Geometry check sheet. Reference: drawing and pictorial views, mm from the part's lowest x, y, z. Give positions to 0.01 mm unless a question says otherwise; leave off trailing zeros. Write each loop counter-clockwise with the first axis right and the second up, starting at its lowest first coordinate (ties: lowest second). Pieces come first, ordered by that corner, then holes. Notation, with made-up numbers: (-14, -12) - (35, -12) arc R6 ccw to (35, -3) - close; hole circle Ø9 at (2.25, 45.25). An arc over 180 degrees is marked (long way). Put each result on its own line as item: value.
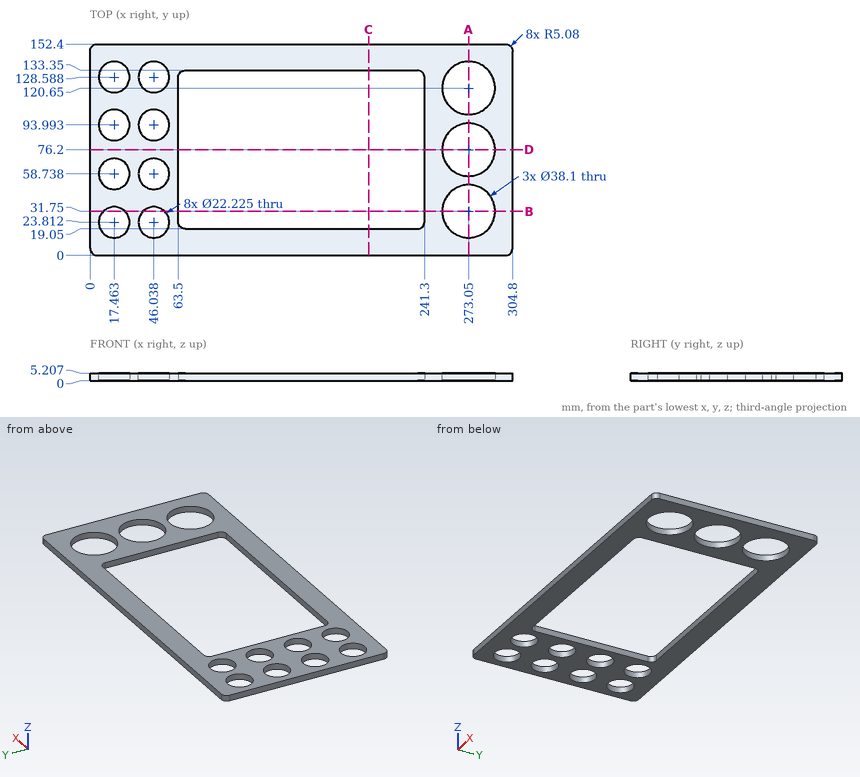
Q1. Section check D-D, the plane y = 76.2. Record the cut outline in (x, z), plus the area to 3 significant figures.
Answers follow:
outline: (0, 0) - (63.5, 0) - (63.5, 5.21) - (0, 5.21) - close; (241.3, 0) - (254, 0) - (254, 5.21) - (241.3, 5.21) - close; (292.1, 0) - (304.8, 0) - (304.8, 5.21) - (292.1, 5.21) - close
area: 463 mm2
Q2. Go/stop test with a flat-tipped pin: pin 1 Ø13.5 at (x, y) = (46.04, 23.81) entering from +Z. Record where the tip stops, or that it passes through.
Answers follow:
pin 1: passes through
Q3. Scan lines: line 1 along X through (y, z) = (25, 1.35) (1 decimal); line 2 along Y through (x, z) = (207.5, 2); line 3 along Y through (x, z) = (43, 1.45). Record each from-to range of solid material in increasing order.
Answers follow:
line 1: x = 0 to 6.4, 28.5 to 35, 57.1 to 63.5, 241.3 to 255.2, 290.9 to 304.8
line 2: y = 0 to 19.05, 133.35 to 152.4
line 3: y = 0 to 13.12, 34.5 to 48.05, 69.43 to 83.3, 104.68 to 117.9, 139.28 to 152.4
Q4. Section check A-A, the plane x = 273.05. Record the cut outline in (y, z).
Answers follow:
outline: (0, 0) - (12.7, 0) - (12.7, 5.21) - (0, 5.21) - close; (50.8, 0) - (57.15, 0) - (57.15, 5.21) - (50.8, 5.21) - close; (95.25, 0) - (101.6, 0) - (101.6, 5.21) - (95.25, 5.21) - close; (139.7, 0) - (152.4, 0) - (152.4, 5.21) - (139.7, 5.21) - close
Q5. Section check B-B, the plane y = 31.75. Record the cut outline in (x, z) (1 decimal).
Answers follow:
outline: (0, 0) - (9.7, 0) - (9.7, 5.2) - (0, 5.2) - close; (25.2, 0) - (38.3, 0) - (38.3, 5.2) - (25.2, 5.2) - close; (53.8, 0) - (63.5, 0) - (63.5, 5.2) - (53.8, 5.2) - close; (241.3, 0) - (254, 0) - (254, 5.2) - (241.3, 5.2) - close; (292.1, 0) - (304.8, 0) - (304.8, 5.2) - (292.1, 5.2) - close
Q6. Section check C-C, the plane x = 201. Record the cut outline in (y, z).
Answers follow:
outline: (0, 0) - (19.05, 0) - (19.05, 5.21) - (0, 5.21) - close; (133.35, 0) - (152.4, 0) - (152.4, 5.21) - (133.35, 5.21) - close
